from build123d import *

# Parameters (mm, degrees)
F1_DEPTH = 22


with BuildPart() as f1:
    # F0 (on Front) → F1 (new body)
    with BuildSketch(Plane.XZ):
        with BuildLine():
            Line((-35.251705, 9.734763), (-44.051705, 9.734763))
            ThreePointArc((-44.051705, 9.734763), (-45.465918, 9.148977), (-46.051705, 7.734763))
            Line((-46.051705, 7.734763), (-46.051705, 6.734763))
            Line((-46.051705, 6.734763), (-54.816158, 6.734763))
            ThreePointArc((-54.816158, 6.734763), (-55.354677, 6.660898), (-55.853418, 6.444761))
            Line((-55.853418, 6.444761), (-60.588965, 3.572245))
            ThreePointArc((-60.588965, 3.572245), (-61.294479, 2.843441), (-61.551705, 1.862248))
            Line((-61.551705, 1.862248), (-61.551705, -4.765237))
            ThreePointArc((-61.551705, -4.765237), (-60.087239, -8.300771), (-56.551705, -9.765237))
            Line((-56.551705, -9.765237), (-12.651705, -9.765237))
            ThreePointArc((-12.651705, -9.765237), (-12.15673, -9.560212), (-11.951705, -9.065237))
            Line((-11.951705, -9.065237), (-11.951705, -7.265237))
            Line((-11.951705, -7.265237), (6.198295, -7.265237))
            Line((6.198295, -7.265237), (6.198295, -9.065237))
            ThreePointArc((6.198295, -9.065237), (6.40332, -9.560212), (6.898295, -9.765237))
            Line((6.898295, -9.765237), (25.448295, -9.765237))
            ThreePointArc((25.448295, -9.765237), (28.983829, -8.300771), (30.448295, -4.765237))
            Line((30.448295, -4.765237), (30.448295, 1.90505))
            ThreePointArc((30.448295, 1.90505), (30.206924, 2.857533), (29.541071, 3.580114))
            Line((29.541071, 3.580114), (25.203537, 6.409828))
            ThreePointArc((25.203537, 6.409828), (24.680792, 6.651809), (24.110761, 6.734763))
            Line((24.110761, 6.734763), (14.948295, 6.734763))
            Line((14.948295, 6.734763), (14.948295, 7.734763))
            ThreePointArc((14.948295, 7.734763), (14.362509, 9.148977), (12.948295, 9.734763))
            Line((12.948295, 9.734763), (7.348295, 9.734763))
            ThreePointArc((7.348295, 9.734763), (5.934082, 9.148977), (5.348295, 7.734763))
            Line((5.348295, 7.734763), (5.348295, 3.734763))
            Line((5.348295, 3.734763), (-10.651705, 3.734763))
            Line((-10.651705, 3.734763), (-10.651705, 7.734763))
            ThreePointArc((-10.651705, 7.734763), (-11.237491, 9.148977), (-12.651705, 9.734763))
            Line((-12.651705, 9.734763), (-18.251705, 9.734763))
            ThreePointArc((-18.251705, 9.734763), (-19.665918, 9.148977), (-20.251705, 7.734763))
            Line((-20.251705, 7.734763), (-20.251705, 7.234763))
            Line((-20.251705, 7.234763), (-33.251705, 7.234763))
            Line((-33.251705, 7.234763), (-33.251705, 7.734763))
            ThreePointArc((-33.251705, 7.734763), (-33.837491, 9.148977), (-35.251705, 9.734763))
        make_face()
        with BuildLine():
            ThreePointArc((-40.90523, -3.219393), (-43.514426, -4.55086), (-46.067619, -3.114923))
            ThreePointArc((-46.067619, -3.114923), (-46.699482, -2.674239), (-47.457145, -2.813521))
            Line((-47.457145, -2.813521), (-49.204705, -3.951495))
            Line((-49.204705, -3.951495), (-56.051705, -3.951495))
            ThreePointArc((-56.051705, -3.951495), (-56.758812, -3.658601), (-57.051705, -2.951495))
            Line((-57.051705, -2.951495), (-57.051705, -0.451495))
            ThreePointArc((-57.051705, -0.451495), (-56.758812, 0.255612), (-56.051705, 0.548505))
            Line((-56.051705, 0.548505), (-49.204805, 0.548505))
            Line((-49.204805, 0.548505), (-47.266027, -0.186586))
            ThreePointArc((-47.266027, -0.186586), (-46.595978, -0.200457), (-46.067649, 0.211886))
            ThreePointArc((-46.067649, 0.211886), (-43.514428, 1.647871), (-40.9052, 0.316361))
            ThreePointArc((-40.9052, 0.316361), (-40.349539, -0.020953), (-39.726865, 0.165639))
            Line((-39.726865, 0.165639), (-38.698705, 1.048505))
            Line((-38.698705, 1.048505), (-22.404805, 1.048505))
            Line((-22.404805, 1.048505), (-21.376582, 0.165586))
            ThreePointArc((-21.376582, 0.165586), (-20.753901, -0.021006), (-20.198239, 0.316318))
            ThreePointArc((-20.198239, 0.316318), (-14.551705, -1.451521), (-20.198269, -3.219265))
            ThreePointArc((-20.198269, -3.219265), (-20.753923, -2.881932), (-21.376606, -3.06851))
            Line((-21.376606, -3.06851), (-25.316505, -6.451495))
            Line((-25.316505, -6.451495), (-35.787205, -6.451495))
            Line((-35.787205, -6.451495), (-39.726916, -3.068671))
            ThreePointArc((-39.726916, -3.068671), (-40.349578, -2.88209), (-40.90523, -3.219393))
        make_face(mode=Mode.SUBTRACT)
        with BuildLine():
            ThreePointArc((14.982149, -3.08637), (9.248661, -1.403859), (15.031143, 0.101673))
            ThreePointArc((15.031143, 0.101673), (15.561388, -0.339456), (16.251102, -0.332352))
            Line((16.251102, -0.332352), (18.345387, 0.4617))
            Line((18.345387, 0.4617), (25.181225, 0.537321))
            ThreePointArc((25.181225, 0.537321), (25.895472, 0.248389), (26.192287, -0.462618))
            Line((26.192287, -0.462618), (26.192287, -2.951495))
            ThreePointArc((26.192287, -2.951495), (25.899394, -3.658601), (25.192287, -3.951495))
            Line((25.192287, -3.951495), (18.345387, -3.951495))
            Line((18.345387, -3.951495), (16.344939, -2.755456))
            ThreePointArc((16.344939, -2.755456), (15.595815, -2.641987), (14.982149, -3.08637))
        make_face(mode=Mode.SUBTRACT)
    extrude(amount=F1_DEPTH)


solid = f1.part
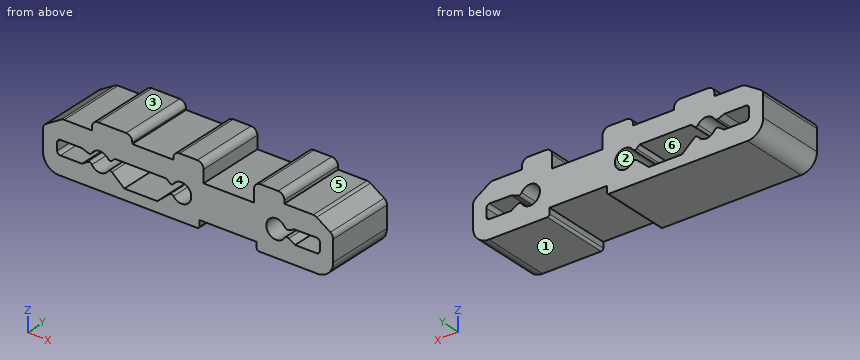
Build history of the part. All positions in model axes, mm. Face numbers are marked on the shaded views. A direction names the side the tool comes from. Round coordinates to 2 decimals unless told otherwise and drop trailing zeros. Loops run counter-clockwise (first coordinate to the right, second up) from the corner with the lowest first, then second, coordinate; pieces in that order, holes last. Notation, with made-up numbers: (-31, -10) -> (-20, -10) arc R14 ccw to (-20, 10) -> close; hole circle Ø2 at (84, 84.25). An arc over 180 degrees is marked (long way). Answer in a Markdown table with one row per item.
Item 1: Saw through at A-A (x = -50). Write the cut outline in (y, z).
Answers below:
| item | result |
|---|---|
| outline | (-22, -9.77) -> (0, -9.77) -> (0, -3.95) -> (-22, -3.95) -> close; (-22, 0.55) -> (0, 0.55) -> (0, 6.73) -> (-22, 6.73) -> close |
Item 2: Which spindle directions (+Z, -Z, +X, -X, +Y, -Y) get a long thin tool onto all of the face, cutting with end or side? Do the marked faces 4, 5 and 6. Say none if no direction does.
Answers below:
| item | result |
|---|---|
| face 4 | +Z, +Y, -Y |
| face 5 | +Z, +X, +Y, -Y |
| face 6 | +Y, -Y |
Item 3: Pin check, flat tips, straight feed: pin 1 (0.5 mm diameter, centred on y = -8, z = -8, fed in from +X); pin 2 (7.5 mm diameter, centred on x = -52, y = -7.5, fed in from +Z); pin 3 (0.9 mm diameter, centred on y = -12.5, z = -8.5, fed in from -X). Stop position of each tip, or through.
Answers below:
| item | result |
|---|---|
| pin 1 | stops at x = 29.46 |
| pin 2 | stops at z = 6.73 |
| pin 3 | stops at x = -60.32 |
Item 4: Saw through at B-B (x = -15.5). Write the cut outline in (y, z).
Answers below:
| item | result |
|---|---|
| outline | (-22, -9.77) -> (0, -9.77) -> (0, -3.68) -> (-22, -3.68) -> close; (-22, 0.78) -> (0, 0.78) -> (0, 9.73) -> (-22, 9.73) -> close |
Item 5: Saw through at D-D (x = -0.5). Write the cut outline in (y, z), and give its area (3 significant figures).
Answers below:
| item | result |
|---|---|
| outline | (-22, -7.27) -> (0, -7.27) -> (0, 3.73) -> (-22, 3.73) -> close |
| area | 242 mm² |
Item 6: Mould opens along Z. For the marked faces 1, 2 and 3 say: +Z half, -Z half, draft (parallel to the pull), parting line (faces both ways), or undercut.
Answers below:
| item | result |
|---|---|
| face 1 | -Z half |
| face 2 | undercut |
| face 3 | +Z half |
Item 7: Saw through at C-C (y = -17.75). State how many separate pieces and enclosed holes the cut face has, and give its area (3 significant figures).
Answers below:
| item | result |
|---|---|
| separate pieces | 1 |
| enclosed holes | 2 |
| area | 1,180 mm² |
Item 8: Drill centre lines: L1, parallel to X at y = -3, z = 7; L2, parallel to X at y = -0.75, z = 8.5; L3, parallel to X at y = -5.25, z = -2. Where is each one in solid material? Low to high. Write a range as [from, to].
Answers below:
| item | result |
|---|---|
| L1 | x = [-46.05, -10.65], [5.35, 14.95] |
| L2 | x = [-45.9, -33.4], [-20.1, -10.8], [5.5, 14.8] |
| L3 | x = [-61.55, -57.05], [-14.6, 9.3], [26.19, 30.45] |
